from build123d import *

# Parameters (mm, degrees)
F1_DEPTH    = 7.5
F2_R        = 5
F3_R        = 10
F4_W        = 6.5123213332
F4_H        = 5.8516720749
F4_R        = 2
F5_DEPTH    = 4
F4_R_2      = 1.5
F6_DEPTH    = 6.5
F7_T1_DEPTH = 21.942419261
F8_R        = 3
F8_R_2      = 1.5
F9_DEPTH    = 1
F10_DEPTH   = 1
F14_DEPTH   = 5


# Not quite as in the source:
# - a fillet or chamfer that OpenCascade refuses, or shapes differently, is made with other operations: its cross-section is extruded or revolved along the edge and cut away or added


with BuildPart() as f1:
    # F0 (on Top) → F1 (new body, symmetric)
    with BuildSketch(Plane.XY):
        Polygon((20, 0), (0, 0), (-20, 0), (-29.3166648167, 3.6331469407), (-30.0432942049, 1.7698139773), (-20.3761671049, -2), (0, -2), (20.3761671049, -2), (30.0432942049, 1.7698139773), (29.3166648167, 3.6331469407), align=None)
    extrude(amount=F1_DEPTH, both=True)

    # F2
    f2_edges = [f1.edges().sort_by_distance(p)[0] for p in [
        (29.67998, 2.70148, 7.5),
        (29.67998, 2.70148, -7.5),
        (-29.67998, 2.70148, 7.5),
        (-29.67998, 2.70148, -7.5),
    ]]
    fillet(f2_edges, radius=F2_R)

    # F3
    f3_edges = [f1.edges().sort_by_distance(p)[0] for p in [
        (20, 0, 0),
        (-20, 0, 0),
        (-20.376167, -2, 0),
        (20.376167, -2, 0),
    ]]
    fillet(f3_edges, radius=F3_R)

    # F4 (on Top) → F5 (join)
    with BuildSketch(Plane.XY):
        with Locations((13.4171620011, -4.9258360375)):
            Rectangle(F4_W, F4_H)
        with Locations((13.4171620011, -5.5516720749)):
            Circle(F4_R, mode=Mode.SUBTRACT)
    extrude(amount=F5_DEPTH)

    # F7: chamfer of 3 on 1 edges, made by hand

    # F7_s2 → F7_t1 (cut)
    with BuildSketch(Plane.YZ.offset(2.4459523706)):
        Polygon((-4.8516720749, 4), (-7.8516720749, 1), (-7.8516720749, 4), align=None)
    extrude(amount=F7_T1_DEPTH, mode=Mode.SUBTRACT)


with BuildPart() as f6:
    # F4 (on Top) → F6 (new body, symmetric)
    with BuildSketch(Plane.XY):
        with Locations((13.4171620011, -5.5516720749)):
            Circle(F4_R_2)
    extrude(amount=F6_DEPTH, both=True)

    # F8 (on face) → F9 (join, symmetric)
    with BuildSketch(Plane.XY.offset(6.5)):
        with Locations((13.4171620011, -5.5516720749)):
            Circle(F8_R)
        with Locations((13.4171620011, -5.5516720749)):
            Circle(F8_R_2, mode=Mode.SUBTRACT)
    extrude(amount=F9_DEPTH, both=True)

    # F10 (add): a face of the model
    f10_faces = [f6.faces().sort_by_distance(p)[0] for p in [
        (10.5020148149, -5.5516720749, 5.5),
    ]]
    extrude(f10_faces, amount=F10_DEPTH)


with BuildPart() as f11_1:
    # F11: instance of F1
    add(f1.part.mirror(Plane.XY))


with BuildPart() as f11_2:
    # F11: instance of F6
    add(f6.part.mirror(Plane.XY))


with BuildPart() as f1_1:
    add(f1.part)

    add(f11_1.part)  # F12 merges F11_1
    # F12: F11_2, F11_1, F6, F1 across plane
    add(f11_2.part.mirror(Plane.YZ))
    add(f11_1.part.mirror(Plane.YZ))
    add(f6.part.mirror(Plane.YZ))
    add(f1.part.mirror(Plane.YZ))

    add(f6.part)  # F14 merges F6
    # F13 (on face) → F14 (join)
    with BuildSketch(Plane.XY.offset(7.5)):
        with BuildLine():
            Line((12.6132123219, -2.5642015695), (12.6032123219, -2.5642015695))
            Line((12.6032123219, -2.5642015695), (12.6032123219, -2.6642015695))
            ThreePointArc((12.6032123219, -2.6642015695), (12.6082111102, -2.6627971285), (12.6132123219, -2.6614013414))
            Line((12.6132123219, -2.6614013414), (12.6132123219, -2.5642015695))
        make_face()
    extrude(amount=-F14_DEPTH)



with BuildPart() as f1_2:
    add(f1_1.part)

    add(f11_2.part)  # F15 merges F11_2
    # F15: F1 across plane
    add(f1_1.part.mirror(Plane.YZ))

    # F16: union 


solid = f1_2.part
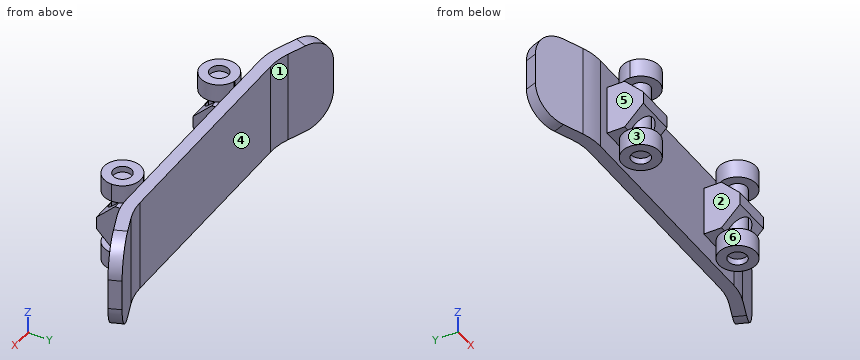
Input: part model. Units: mm. Frame: model coordinates. Face numbers are marked on the shaded views. A direction names the side the tool comes from. Round coordinates to 2 decimals unless told otherwise and drop trailing zeros. Write each loop counter-clockwise with the first axis right and the second up, starting at its lowest first coordinate (ties: lowest second). Pieces come first, ordered by that corner, then holes.
1) Contact query for flat-ended pins moving along their axis: P1, Ø3, axis at y = -6, z = 1, coming from the -X side; P2, Ø2, axis at x = -12.5, z = 0.5, coming from the -Y side; P3, Ø0.9, axis at x = 13, y = -5, coming from the -Z side; P4, Ø4, axis at y = 0.5, z = -4, coming from the -X side. Output: stop coordinate, or through.
2) Cut plane A-A (z = 5.5). Count the separate pieces of the cut face and the enclosed holes in it, then the cut area to 3 significant figures.
3) Cut plane C-C (x = -5). Return the cut outline in (y, z).
4) Draft query along Y for the marked faces 4, 5 and 6. Return one class per face: pulls with the +Y half, pulls with the -Y half, needs draft (parallel to the pull), parting line crosses it, or undercut.
5) Reachability of the marked faces 1, 2 and 3 from +Z, -Z, +X, -X, +Y, -Y: full face, straight path, thin tool, end or side. Return the list, or none.
6) Ray query, L1, parallel to Z at x = 14, y = -3; L2, parallel to X at y = -6.5, z = -0.25; L3, parallel to Y at x = 11, z = 0.75. Return the intervals inside material, ascending.
Geometry says:
1. P1: stops at x = -16.67
1. P2: stops at y = -7.85
1. P3: stops at z = -6.5
1. P4: stops at x = -30.04
2. separate pieces: 3
2. enclosed holes: 0
2. area: 174 mm2
3. outline: (-2, -7.5) - (0, -7.5) - (0, 7.5) - (-2, 7.5) - close
4. face 4: pulls with the +Y half
4. face 5: needs draft
4. face 6: undercut
5. face 1: +Z, -Z, +Y
5. face 2: +Z, -Z, -Y
5. face 3: -Z
6. L1: z = -7.5 to -4.5, -4 to 4, 4.5 to 7.5
6. L2: x = -16.67 to -15.18, -14.58 to -12.25, -11.66 to -10.16, 10.16 to 11.66, 12.25 to 14.58, 15.18 to 16.67
6. L3: y = -7.85 to 0
